For this review, use the dimensioned drawing (mm, ordinates from the lowest corner) and the shaded views. A direction names the side the tool comes from. Coordinates: 2 decimals unless noted, no trailing zeros. Loops run counter-clockwise (first coordinate to the right, second up) from the corner with the lowest first, then second, coordinate; pieces in that order, holes last. Notation, with made-up numbers: M 42,-14.5 L 50,-14.5 A21 cw 50,14.5 Z; hole C 45.25,-15 d9. An arc over 180 degrees is marked long. Write item = value, one per line. Start each with the question number.
Q1. We need section A-A on z = 14.5. Give the boundary of the cut face in (x, y), and give its area (3 significant figures).
Q2. Clearance check with flat-ended pins moving along their axes: pin 1 Ø1.5 at (y, z) = (3.5, 13) entering from -X; pin 2 Ø1 at (y, z) = (7, 18.5) entering from -X; pin 3 Ø1.5 at (x, y) = (14.5, 1.5) entering from -Z. State where each tip first meets the part, or that it passes through.
Q3. We need section D-D on z = 2. Give the boundary of the cut face in (x, y), and give its area (3 significant figures).
Q4. For the marked faces 1 and 2, list the 3-axis set-ups (+Z, -Z, +X, -X, +Y, -Y) from which the entire face can be reached by the end or side of a thin tool; tool diameter is ignored.
Q5. Mouldability with a two-part tool opening along X and no side actions: class the marked faces 3 and 4 as released by +X, released by -X, zero draft, split by the parting line, or undercut.
Q6. We need section B-B on x = 10. Give the boundary of the cut face in (y, z), and give its area (4 significant figures).
Q7. Wall thickness on probe 1 along Z at (x, y) = (2, 5.15); probe 2 along Y at (x, z) = (22, 8.75); probe 3 along Z at (x, y) = (10, 3): over which ranges is each line inside the solid? List them lowest first.
Q8. We need section C-C on z = 19.5. Give the boundary of the cut face in (x, y).
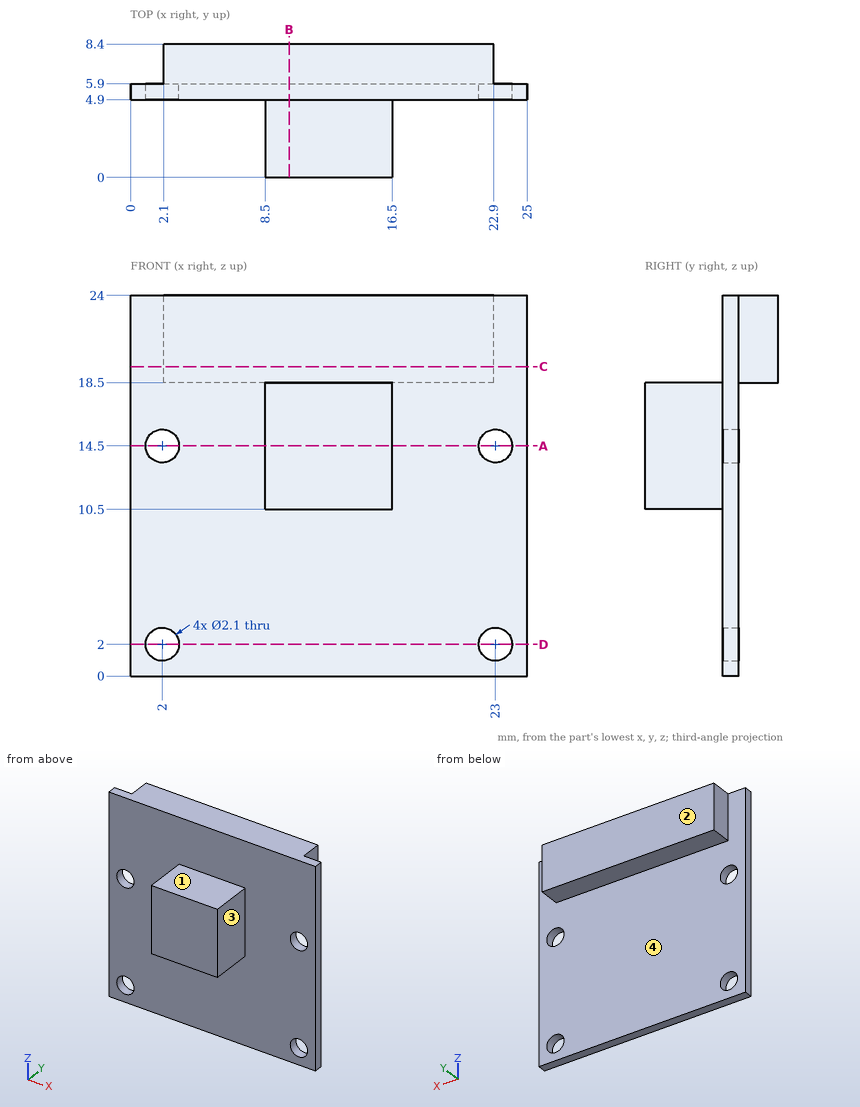
Returned:
q1.outline = M 0,4.9 L 0.95,4.9 L 0.95,5.9 L 0,5.9 Z; M 3.05,4.9 L 8.5,4.9 L 8.5,0 L 16.5,0 L 16.5,4.9 L 21.95,4.9 L 21.95,5.9 L 3.05,5.9 Z; M 24.05,4.9 L 25,4.9 L 25,5.9 L 24.05,5.9 Z
q1.area = 60.0 mm^2
q2.pin_1 = 8.5
q2.pin_2 = 2.1
q2.pin_3 = 10.5
q3.outline = M 0,4.9 L 0.95,4.9 L 0.95,5.9 L 0,5.9 Z; M 3.05,4.9 L 21.95,4.9 L 21.95,5.9 L 3.05,5.9 Z; M 24.05,4.9 L 25,4.9 L 25,5.9 L 24.05,5.9 Z
q3.area = 20.8 mm^2
q4.face_1 = +Z, +X, -X, -Y
q4.face_2 = +Z, -Z, +X, -X, +Y
q5.face_3 = released by +X
q5.face_4 = zero draft
q6.outline = M 0,10.5 L 4.9,10.5 L 4.9,0 L 5.9,0 L 5.9,18.5 L 8.4,18.5 L 8.4,24 L 4.9,24 L 4.9,18.5 L 0,18.5 Z
q6.area = 76.95 mm^2
q7.probe_1 = 0 to 0.95, 3.05 to 13.45, 15.55 to 24
q7.probe_2 = 4.9 to 5.9
q7.probe_3 = 10.5 to 18.5
q8.outline = M 0,4.9 L 25,4.9 L 25,5.9 L 22.9,5.9 L 22.9,8.4 L 2.1,8.4 L 2.1,5.9 L 0,5.9 Z
